from build123d import *

# Parameters (mm, degrees)
F0_W     = 22.86
F0_H     = 22.86
F1_DEPTH = 67.31
F2_W     = 22.86
F2_H     = 22.86
F3_DEPTH = 12.7508
F8_T     = -2.54


with BuildPart() as f1:
    # F0 (on Top) → F1 (new body)
    with BuildSketch(Plane.XY):
        Rectangle(F0_W, F0_H)
    extrude(amount=F1_DEPTH)

    # F2 (on face) → F3 (join)
    with BuildSketch(Plane.XY.offset(67.31)):
        Rectangle(F2_W, F2_H)
    extrude(amount=F3_DEPTH)

    # F4 (on Right) → F5 (revolve, cut)
    with BuildSketch(Plane.YZ):
        Polygon((0, -11.43), (0, 67.31), (-5.08, 67.31), (-3.429, -11.43), align=None)
    revolve(axis=Axis((0, 0, 27.94), (0, 0, -1)), mode=Mode.SUBTRACT)

    # F6 (on Right) → F7 (revolve, cut)
    with BuildSketch(Plane.YZ):
        with BuildLine():
            Line((0, 83.82), (0, 67.31))
            Line((0, 67.31), (6.35, 67.31))
            ThreePointArc((6.35, 67.31), (9.0440768363, 68.4259231637), (10.16, 71.12))
            Line((10.16, 71.12), (10.16, 80.01))
            ThreePointArc((10.16, 80.01), (9.0440768363, 82.7040768363), (6.35, 83.82))
            Line((6.35, 83.82), (0, 83.82))
        make_face()
    revolve(axis=Axis((0, 0, 75.565), (0, 0, 1)), mode=Mode.SUBTRACT)

    # F8
    f8_openings = [f1.faces().sort_by_distance(p)[0] for p in [
        (0, -11.106711, 0),
    ]]
    offset(amount=F8_T, openings=f8_openings)


solid = f1.part
Design review of the part built by this model. Coordinates are the model's own, in mm. A direction names the side the tool comes from. Coordinates: 2 decimals unless noted, no trailing zeros. Order: outer loops, then holes, each group sorted by start corner. A loop starts at its lowest first (then second) coordinate and runs counter-clockwise, first axis right, second up.
Item 1: Take a section at A-A, the plane z = 12. Write out the cut boundary in (x, y), then the cut area to 3 significant figures.
Item 2: Take a section at C-C, the plane z = 63.5. Write out the cut boundary in (x, y), then the cut area to 3 significant figures.
Item 3: Take a section at B-B, the plane z = 75.5. Write out the cut boundary in (x, y).
Item 4: For pin 1 Ø10 at (x, y) = (2.5, 0.5) entering from +Z, flat-tipped, find the tip position at first contact; note if it passes through.
Item 5: For line 1 (X direction, y = 0, z = 73); line 2 (Y direction, x = 0.5, z = 14); line 3 (Y direction, x = 3.25, z = 11), list the stretches that pass through material, from the lowest coordinate up.
Item 6: The part is to be moulded in two halves that separate along Y. For faces 4 (the flat face through (-11.43, 0, 39)), 5 (the flat face through (0, 11.43, 39)), 6 (the flat face through (0, -8.89, 34)), say which applies: pulls with the +Y half, pulls with the -Y half, needs draft (parallel to the pull), parting line crosses it, or undercut.
Item 7: For faces 1 (the flat face through (11.43, 0, 39)), 2 (the conical face through (4.26, 0.95, 33.18)), 3 (the flat face through (0, 8.89, 34)), list the 3-axis set-ups (+Z, -Z, +X, -X, +Y, -Y) from which the entire face can be reached by the end or side of a thin tool; tool diameter is ignored.
The answers:
1. outline: (-11.43, -11.43) - (11.43, -11.43) - (11.43, 11.43) - (-11.43, 11.43) - close; circle Ø12.92 at (0, 0); hole (-8.89, -8.89) - (8.89, -8.89) - (8.89, 8.89) - (-8.89, 8.89) - close; hole circle Ø7.84 at (0, 0)
1. area: 289 mm2
2. outline: (-11.43, -11.43) - (11.43, -11.43) - (11.43, 11.43) - (-11.43, 11.43) - close; circle Ø15.08 at (0, 0); hole (-8.89, -8.89) - (8.89, -8.89) - (8.89, 8.89) - (-8.89, 8.89) - close; hole circle Ø10 at (0, 0)
2. area: 307 mm2
3. outline: (-11.43, -11.43) - (11.43, -11.43) - (11.43, 11.43) - (-11.43, 11.43) - close; hole circle Ø20.32 at (0, 0)
4. pin 1: stops at z = 67.5
5. line 1: x = -11.43 to -10.16, 10.16 to 11.43
5. line 2: y = -11.43 to -8.89, -6.48 to -3.93, 3.93 to 6.48, 8.89 to 11.43
5. line 3: y = -11.43 to -8.89, -5.56 to -2.15, 2.15 to 5.56, 8.89 to 11.43
6. face 4: needs draft
6. face 5: pulls with the +Y half
6. face 6: undercut
7. face 1: +Z, -Z, +X, +Y, -Y
7. face 2: +Z
7. face 3: -Z
